Autodesk Inventor part; units mm, degrees
ref_plane "YZ Plane" through (0, 0, 0) normal (1, 0, 0) x (0, 1, 0)
ref_plane "XZ Plane" through (0, 0, 0) normal (0, 1, 0) x (-1, 0, 0)
ref_plane "XY Plane" through (0, 0, 0) normal (0, 0, 1) x (1, 0, 0)
sketch "Esboço1" plane through (0, 0, 0) normal (0, 0, 1) x (1, 0, 0)
  line L0 (-215, -42) -> (215, -42)
  line L1 (215, -42) -> (215, 42)
  line L2 (215, 42) -> (-215, 42)
  line L3 (-215, 42) -> (-215, -42)
  point P0 (0, 0)
  dimension "d2" = 430
  dimension "d4" = 84
  dimension "d6" = 215
  dimension "d7" = 42
extrude "Extrusão1" add sketch "Esboço1" against normal blind 4
sketch "Esboço3" plane through (0, 0, 0) normal (0, 0, 1) x (1, 0, 0)
  line L0 (-215, -42) -> (-215, 42)
  line L1 (215, -42) -> (-215, -42)
  line L2 (-215, 37) -> (215, 37) construction
  line L3 (-210, 42) -> (-210, -42) construction
  line L4 (210, 42) -> (210, -42) construction
  line L5 (-215, -37) -> (215, -37) construction
  line L6 (-8, 37) -> (-8, -37) construction
  line L7 (8, 37) -> (8, -37) construction
  line L8 (210, 37) -> (210, -37)
  line L9 (-202, 37) -> (-202, -37)
  line L10 (-16, 37) -> (-16, -37)
  line L11 (-117, 37) -> (-117, -37)
  line L12 (-101, 37) -> (-101, -37)
  line L13 (16, 37) -> (16, -37)
  line L14 (202, 37) -> (202, -37)
  line L15 (101, 37) -> (101, -37)
  line L16 (117, 37) -> (117, -37)
  line L17 (-202, -37) -> (-117, -37)
  line L18 (-202, 37) -> (-117, 37)
  line L19 (-101, 37) -> (-16, 37)
  line L20 (-16, -37) -> (-101, -37)
  line L21 (202, 37) -> (117, 37)
  line L22 (101, 37) -> (16, 37)
  line L23 (-215, 42) -> (215, 42)
  line L24 (16, -37) -> (101, -37)
  line L25 (117, -37) -> (202, -37)
  point P0 (0, 0)
  dimension "d79" = 79
  dimension "d80" = 5
  dimension "d81" = 79
  dimension "d82" = 5
  dimension "d83" = 79
  dimension "d84" = 5
  dimension "d85" = 79
  dimension "d86" = 5
  dimension "d87" = 199
  dimension "d88" = 114
  dimension "d89" = 98
  dimension "d90" = 13
  dimension "d91" = 79
  dimension "d92" = 5
  dimension "d93" = 425
  dimension "d94" = 417
  dimension "d95" = 332
  dimension "d96" = 316
  dimension "d97" = 231
  dimension "d98" = 223
  dimension "d99" = 207
  dimension "d100" = 5
  dimension "d101" = 430
  dimension "d102" = 430
  dimension "d103" = 84
  dimension "d104" = 84
extrude "Extrusão2" cut sketch "Esboço3" against normal blind 10
sketch "Esboço5" plane through (0, 0, -4) normal (0, 0, -1) x (-1, 0, 0)
  line L0 (-215, 37) -> (215, 37) construction
  line L1 (-210, 42) -> (-210, -42) construction
  line L2 (210, 42) -> (210, -42) construction
  line L3 (-215, -37) -> (215, -37) construction
  line L4 (-8, 37) -> (-8, -37) construction
  line L5 (8, 37) -> (8, -37) construction
  line L6 (-117, -37) -> (-202, -37)
  line L7 (-202, -37) -> (-210, -37)
  line L8 (-210, 37) -> (-210, -37)
  line L9 (-210, 37) -> (-202, 37)
  line L10 (-202, 37) -> (-117, 37)
  line L11 (-202, 37) -> (-202, -37)
  line L12 (-101, 37) -> (-16, 37)
  line L13 (-117, 37) -> (-101, 37)
  line L14 (-101, -37) -> (-101, 37)
  line L15 (-101, 37) -> (-101, -37)
  line L16 (-101, -37) -> (-117, -37)
  line L17 (-117, 37) -> (-117, -37)
  line L18 (-16, 37) -> (-8, 37)
  line L19 (-8, 37) -> (-8, -37)
  line L20 (-8, -37) -> (-16, -37)
  line L21 (-16, 37) -> (-16, -37)
  line L22 (-16, -37) -> (-16, 37)
  line L23 (16, 37) -> (101, 37)
  line L24 (8, 37) -> (16, 37)
  line L25 (16, -37) -> (16, 37)
  line L26 (16, 37) -> (16, -37)
  line L27 (16, -37) -> (8, -37)
  line L28 (8, 37) -> (8, -37)
  line L29 (101, 37) -> (101, -37)
  line L30 (101, 37) -> (117, 37)
  line L31 (117, -37) -> (117, 37)
  line L32 (117, 37) -> (117, -37)
  line L33 (117, -37) -> (101, -37)
  line L34 (101, -37) -> (101, 37)
  line L35 (117, 37) -> (202, 37)
  line L36 (202, 37) -> (210, 37)
  line L37 (210, -37) -> (210, 37)
  line L38 (202, -37) -> (117, -37)
  line L39 (202, 37) -> (202, -37)
  line L40 (202, -37) -> (210, -37)
  point P0 (0, 0)
  point P1 (0, 0)
  point P2 (0, 0)
  dimension "d188" = 109
  dimension "d189" = 109
  dimension "d190" = 125
  dimension "d191" = 327
  dimension "d192" = 98
  dimension "d193" = 98
  dimension "d194" = 79
  dimension "d195" = 5
  dimension "d196" = 37
  dimension "d197" = 117
  dimension "d198" = 79
  dimension "d199" = 5
  dimension "d200" = 332
  dimension "d201" = 332
  dimension "d202" = 90
  dimension "d203" = 90
  dimension "d204" = 90
  dimension "d205" = 90
  dimension "d206" = 8
  dimension "d207" = 93
  dimension "d208" = 194
  dimension "d209" = 226
  dimension "d210" = 311
  dimension "d211" = 327
  dimension "d212" = 412
  dimension "d213" = 74
  dimension "d214" = 210
  dimension "d215" = 37
  dimension "d216" = 74
  dimension "d217" = 210
  dimension "d218" = 37
extrude "Extrusão4" cut sketch "Esboço5" against normal blind 2
sketch "Esboço6" plane through (0, 0, -2) normal (0, 0, -1) x (-1, 0, 0)
  line L0 (-210, 37) -> (-202, 37)
  line L1 (-210, 37) -> (-8, 37)
  line L2 (-210, -37) -> (-210, 37)
  line L3 (-210, 18.5) -> (210, 18.5) construction
  line L4 (210, 37) -> (210, -37)
  line L5 (-210, -18.5) -> (210, -18.5) construction
  line L6 (-117, 37) -> (-101, 37)
  line L7 (-206, 37) -> (-206, -37) construction
  line L8 (-113, 37) -> (-113, -37) construction
  line L9 (-105, 37) -> (-105, -37) construction
  line L10 (8, 37) -> (16, 37)
  line L11 (12, 37) -> (12, -37) construction
  line L12 (-16, 37) -> (-8, 37)
  line L13 (-12, 37) -> (-12, -37) construction
  line L14 (-8, -37) -> (-16, -37)
  line L15 (101, 37) -> (117, 37)
  line L16 (105, 37) -> (105, -37) construction
  line L17 (113, 37) -> (113, -37) construction
  line L18 (202, 37) -> (210, 37)
  line L19 (206, 37) -> (206, -37) construction
  line L20 (210, -37) -> (8, -37)
  point P0 (0, 0)
  point P1 (-206, 18.5)
  point P2 (-206, -18.5)
  point P3 (-113, -18.5)
  point P4 (-105, -18.5)
  point P5 (-113, 18.5)
  point P6 (-105, 18.5)
  point P7 (-12, 18.5)
  point P8 (-12, -18.5)
  point P9 (12, -18.5)
  point P10 (12, 18.5)
  point P11 (105, 18.5)
  point P12 (113, 18.5)
  point P13 (113, -18.5)
  point P14 (105, -18.5)
  point P15 (206, 18.5)
  point P16 (206, -18.5)
  dimension "d230" = 18.5
  dimension "d231" = 55.5
  dimension "d232" = 97
  dimension "d233" = 105
  dimension "d234" = 315
  dimension "d235" = 323
  dimension "d236" = 416
  dimension "d237" = 0
  dimension "d238" = 0
  dimension "d239" = 0
  dimension "d240" = 0
  dimension "d241" = 74
  dimension "d242" = 0
hole "Furo1" at (206, 18.5, -2) at (206, -18.5, -2) at (113, -18.5, -2) at (105, -18.5, -2) at (113, 18.5, -2) at (105, 18.5, -2) at (12, 18.5, -2) at (12, -18.5, -2) at (-12, -18.5, -2) at (-12, 18.5, -2) at (-105, 18.5, -2) at (-113, 18.5, -2) at (-113, -18.5, -2) at (-105, -18.5, -2) at (-206, 18.5, -2) at (-206, -18.5, -2) direction (0, 0, 1) diameter 2.459 end through all
equation "\"d2\" = 2 * d6"
equation "\"d4\" = 2 * d7"
properties part number "Ra-Manager_Painel_Traseiro" material "Aço, carbono"
Design review of the part built by this model. Coordinates are the model's own, in mm. A direction names the side the tool comes from. Coordinates: 2 decimals unless noted, no trailing zeros. Order: outer loops, then holes, each group sorted by start corner. A loop starts at its lowest first (then second) coordinate and runs counter-clockwise, first axis right, second up. Notation, with made-up numbers: (-40, 5.5) - (2, 5.5) arc R13 ccw to (2, 10.5) - close; hole circle Ø9 at (-15, 83.5). An arc over 180 degrees is marked (long way). One line per question, with ' | ' between items.
Q1. Clearance check with flat-ended pins moving along their axes: pin 1 Ø8 at (x, y) = (111, -8.5) entering from -Z; pin 2 Ø4 at (x, y) = (113, -18.5) entering from +Z. State where each tip first meets the part, or that it passes through.
Answer key:
pin 1: stops at z = -2 | pin 2: stops at z = 0
Q2. For faces 1 (the flat face through (109, 1, -2)), 2 (the flat face through (-1, -3, -4)), list the 3-axis set-ups (+Z, -Z, +X, -X, +Y, -Y) from which the entire face can be reached by the end or side of a thin tool; tool diameter is ignored.
Answer key:
face 1: -Z | face 2: -Z, +X, -X, +Y, -Y
Q3. Consider section A-A, the plane y = -8.5. Give the boundary of the cut face in (x, z).
Answer key:
outline: (-215, -4) - (-210, -4) - (-210, -2) - (-202, -2) - (-202, 0) - (-215, 0) - close; (-117, -2) - (-101, -2) - (-101, 0) - (-117, 0) - close; (-16, -2) - (-8, -2) - (-8, -4) - (8, -4) - (8, -2) - (16, -2) - (16, 0) - (-16, 0) - close; (101, -2) - (117, -2) - (117, 0) - (101, 0) - close; (202, -2) - (210, -2) - (210, -4) - (215, -4) - (215, 0) - (202, 0) - close
Q4. Consider section B-B, the plane x = 156. Give the boundary of the cut face in (y, z), then the cut area to 3 significant figures.
Answer key:
outline: (-42, -4) - (-37, -4) - (-37, 0) - (-42, 0) - close; (37, -4) - (42, -4) - (42, 0) - (37, 0) - close | area: 40.0 mm2
Q5. The part is to be moulded in two halves that separate along X. For faces 3 (the flat face through (-206, 1, -2)), 4 (the flat face through (-1, -3, 0)), say which applies: +X half, -X half, draft (parallel to the pull), parting line (faces both ways), or undercut.
Answer key:
face 3: undercut | face 4: draft
Q6. To check wall thickness, follow line 1 along X through (y, z) = (6.5, -1.6); line 2 along X through (y, z) = (-14, -2.95); line 3 along Y through (x, z) = (206, -1.3). State the ranges of each line that lie inside material, in increasing order.
Answer key:
line 1: x = -215 to -202, -117 to -101, -16 to 16, 101 to 117, 202 to 215 | line 2: x = -215 to -210, -8 to 8, 210 to 215 | line 3: y = -42 to -19.73, -17.27 to 17.27, 19.73 to 42
